Here's how the part is built. I have some questions about the finished solid (model axes, mm). Face numbers are marked on the shaded views. A direction names the side the tool comes from. Round coordinates to 2 decimals unless told otherwise and drop trailing zeros. Loops run counter-clockwise (first coordinate to the right, second up) from the corner with the lowest first, then second, coordinate; pieces in that order, holes last. Notation, with made-up numbers: (83.5, -5) - (87.5, -5) arc R7 ccw to (87.5, 8) - close; hole circle Ø7 at (81.5, -25). An arc over 180 degrees is marked (long way). Answer as a JSON object with one key per item and string values. Group by question number.
1) If I drill on line 1 along X through (y, z) = (-9, 19); line 2 along Z through (x, y) = (32, -27.5); line 3 along Z through (x, y) = (-10, 6), over which ranges is the centre line in solid material (lowest first)? Write a range as [from, to].
2) I want a section at B-B, the plane z = 15.5. Please give me the cut outline in (x, y), then the cut area to 3 significant figures.
3) I want a section at A-A, the plane x = -7. Please give me the cut outline in (y, z).
4) I want a section at D-D, the plane y = 0.5. Please give me the cut outline in (x, z), then the cut area to 3 significant figures.
5) Will these pins go through, and if not, where does the flat tip stop? P1, Ø7, axis at x = -19.24, y = -30.49, coming from the +Z side; P2, Ø5, axis at x = 24, y = 0, coming from the +Z side; P3, Ø3, axis at y = -27.5, z = 22, coming from the +X side.
6) I want a section at C-C, the plane y = -25.5. Please give me the cut outline in (x, z).
7) Which directions (+Z, -Z, +X, -X, +Y, -Y) give clear straight access to the entire face, cutting with the end or side of a thin tool? Please do the marked faces 4, 5 and 6.
8) If we mould it in two halves opening along X, with no side actions, what happens to the marked faces 1, 2 and 3? For each: pulls with the +X half, pulls with the -X half, needs draft (parallel to the pull), parting line crosses it, or undercut.
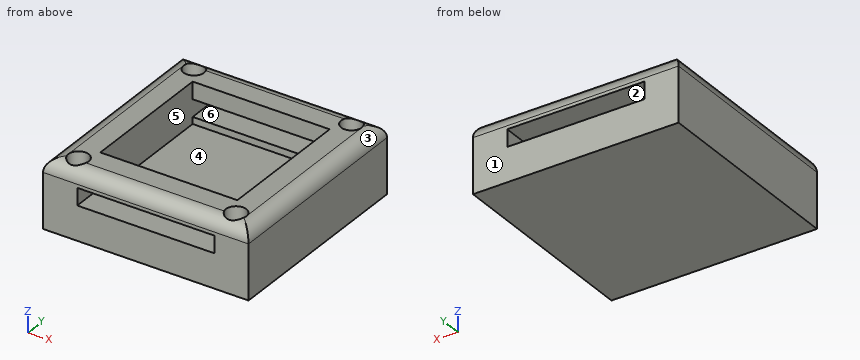
from build123d import *

# Parameters (mm, degrees)
F0_W        = 76.2
F0_H        = 76.2
F1_DEPTH    = 25.4
F2_W        = 50.8
F2_H        = 6.35
F3_DEPTH    = 76.201
F4_W        = 50.8
F4_H        = 50.8
F5_DEPTH    = 15.24
F6_R        = 3.81
F7_DEPTH    = 5.08
F8_T1_DEPTH = 101.6
F8_T3_DEPTH = 101.6


# Not quite as in the source:
# - a fillet or chamfer that OpenCascade refuses, or shapes differently, is made with other operations: its cross-section is extruded or revolved along the edge and cut away or added


with BuildPart() as f1:
    # F0 (on Top) → F1 (new body)
    with BuildSketch(Plane.XY):
        with Locations((9.967116639, 1.2604303423)):
            Rectangle(F0_W, F0_H)
    extrude(amount=F1_DEPTH)

    # F2 (on face) → F3 (cut, through all)
    with BuildSketch(Plane.XZ.offset(36.8395696577)):
        with Locations((9.967116639, 15.875)):
            Rectangle(F2_W, F2_H)
    extrude(amount=-F3_DEPTH, mode=Mode.SUBTRACT)

    # F4 (on face) → F5 (cut)
    with BuildSketch(Plane.XY.offset(25.4)):
        with Locations((9.967116639, 1.2604303423)):
            Rectangle(F4_W, F4_H)
    extrude(amount=-F5_DEPTH, mode=Mode.SUBTRACT)

    # F6 (on face) → F7 (cut)
    with BuildSketch(Plane.XY.offset(25.4)):
        with Locations((-19.242883361, 33.0104303423)):
            Circle(F6_R)
        with Locations((39.177116639, 33.0104303423)):
            Circle(F6_R)
        with Locations((-19.242883361, -30.4895696577)):
            Circle(F6_R)
        with Locations((39.177116639, -30.4895696577)):
            Circle(F6_R)
    extrude(amount=-F7_DEPTH, mode=Mode.SUBTRACT)

    # F8: fillet of radius 5.08 on 4 edges, made by hand

    # F8_s2 → F8_t1 (cut)
    with BuildSketch(Plane.XZ.offset(-52.0604303423)):
        with BuildLine():
            ThreePointArc((48.067116639, 20.32), (46.5792190874, 23.9121024484), (42.987116639, 25.4))
            Line((42.987116639, 25.4), (48.067116639, 25.4))
            Line((48.067116639, 25.4), (48.067116639, 20.32))
        make_face()
        with BuildLine():
            ThreePointArc((-23.052883361, 25.4), (-26.6449858094, 23.9121024484), (-28.132883361, 20.32))
            Line((-28.132883361, 20.32), (-28.132883361, 25.4))
            Line((-28.132883361, 25.4), (-23.052883361, 25.4))
        make_face()
    extrude(amount=F8_T1_DEPTH, mode=Mode.SUBTRACT)

    # F8_s4 → F8_t3 (cut)
    with BuildSketch(Plane.YZ.offset(-40.832883361)):
        with BuildLine():
            ThreePointArc((-31.7595696577, 25.4), (-35.3516721061, 23.9121024484), (-36.8395696577, 20.32))
            Line((-36.8395696577, 20.32), (-36.8395696577, 25.4))
            Line((-36.8395696577, 25.4), (-31.7595696577, 25.4))
        make_face()
        with BuildLine():
            ThreePointArc((39.3604303423, 20.32), (37.8725327907, 23.9121024484), (34.2804303423, 25.4))
            Line((34.2804303423, 25.4), (39.3604303423, 25.4))
            Line((39.3604303423, 25.4), (39.3604303423, 20.32))
        make_face()
    extrude(amount=F8_T3_DEPTH, mode=Mode.SUBTRACT)


solid = f1.part
Outcome:
{
 "1": {"line 1": "[-28.13, -15.43], [35.37, 48.07]", "line 2": "[0, 12.7], [19.05, 25.4]", "line 3": "[0, 10.16]"},
 "2": {"outline": "(-28.13, -36.84) - (-15.43, -36.84) - (-15.43, 39.36) - (-28.13, 39.36) - close; (35.37, -36.84) - (48.07, -36.84) - (48.07, 39.36) - (35.37, 39.36) - close", "area": "1,940 mm^2"},
 "3": {"outline": "(-36.84, 0) - (39.36, 0) - (39.36, 12.7) - (26.66, 12.7) - (26.66, 10.16) - (-24.14, 10.16) - (-24.14, 12.7) - (-36.84, 12.7) - close; (-36.84, 19.05) - (-24.14, 19.05) - (-24.14, 25.4) - (-31.76, 25.4) arc R5.08 ccw to (-36.84, 20.32) - close; (26.66, 19.05) - (39.36, 19.05) - (39.36, 20.32) arc R5.08 ccw to (34.28, 25.4) - (26.66, 25.4) - close"},
 "4": {"outline": "(-28.13, 0) - (48.07, 0) - (48.07, 20.32) arc R5.08 ccw to (42.99, 25.4) - (35.37, 25.4) - (35.37, 10.16) - (-15.43, 10.16) - (-15.43, 25.4) - (-23.05, 25.4) arc R5.08 ccw to (-28.13, 20.32) - close", "area": "1,150 mm^2"},
 "5": {"P1": "z = 20.32", "P2": "z = 10.16", "P3": "x = 48.06"},
 "6": {"outline": "(-28.13, 0) - (48.07, 0) - (48.07, 20.32) arc R5.08 ccw to (42.99, 25.4) - (-23.05, 25.4) arc R5.08 ccw to (-28.13, 20.32) - close; hole (-15.43, 12.7) - (35.37, 12.7) - (35.37, 19.05) - (-15.43, 19.05) - close"},
 "7": {"face 4": "+Z", "face 5": "none", "face 6": "+Y, -Y"},
 "8": {"face 1": "needs draft", "face 2": "undercut", "face 3": "pulls with the +X half"}
}
